Autodesk Inventor part; units mm, degrees
ref_plane "YZ Plane" through (0, 0, 0) normal (1, 0, 0) x (0, 1, 0)
ref_plane "XZ Plane" through (0, 0, 0) normal (0, 1, 0) x (-1, 0, 0)
ref_plane "XY Plane" through (0, 0, 0) normal (0, 0, 1) x (1, 0, 0)
sketch "Boceto1" plane through (0, 0, 0) normal (0, 1, 0) x (-1, 0, 0)
  circle A0 centre (22.76, 7.95) radius 1.5
  circle A1 centre (-26.24, 7.95) radius 1.5
  line L0 (29.635, -14.19) -> (29.635, 11.2)
  line L1 (29.635, 11.2) -> (-33.115, 11.2)
  line L2 (-33.115, 11.2) -> (-33.115, -14.19)
  line L3 (-33.115, -14.19) -> (29.635, -14.19)
  line L4 (-1.74, -3.0983) -> (-1.74, -1.495)
  line L5 (-1.74, -1.495) -> (-3.5727, -1.495)
  circle A2 centre (26.385, -10.94) radius 1.5
  circle A3 centre (-29.865, -10.94) radius 1.5
  circle A4 centre (26.385, 7.95) radius 1.5
  circle A5 centre (-29.865, 7.95) radius 1.5
  dimension "d5" = 25.39
  dimension "d6" = 62.75
  dimension "d7" = 3
  dimension "d8" = 3.25
  dimension "d9" = 3.25
  dimension "d10" = 49
  dimension "d11" = 0
  dimension "d24" = 3
extrude "Extrusión1" add sketch "Boceto1" along normal blind 3
sketch "Boceto2" plane through (0, 3, 0) normal (0, 1, 0) x (1, 0, 0)
  circle A0 centre (-26.385, -7.95) radius 1.5
  circle A1 centre (-26.385, -7.95) radius 2.5
  circle A2 centre (-26.385, 10.94) radius 1.5
  circle A3 centre (-26.385, 10.94) radius 2.5
  circle A4 centre (29.865, 10.94) radius 1.5
  circle A5 centre (29.865, 10.94) radius 2.5
  circle A6 centre (29.865, -7.95) radius 1.5
  circle A7 centre (29.865, -7.95) radius 2.5
  point P0 (0, 0)
  dimension "d14" = 5
  dimension "d15" = 5
  dimension "d16" = 5
  dimension "d17" = 5
extrude "Extrusión2" add sketch "Boceto2" along normal blind 3
sketch "Boceto3" plane through (0, 0, 0) normal (0, -1, 0) x (1, 0, 0)
  circle A0 centre (-22.76, 7.95) radius 1.5
  circle A1 centre (-22.76, 7.95) radius 3
  circle A2 centre (26.24, 7.95) radius 1.5
  circle A3 centre (26.24, 7.95) radius 3
  point P0 (0, 0)
  dimension "d20" = 6
  dimension "d21" = 6
extrude "Extrusión3" add sketch "Boceto3" along normal blind 15
properties part number "Soporte 16 pwm"
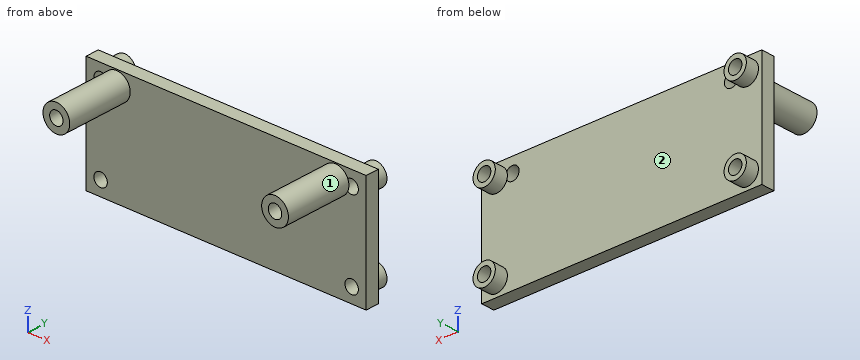
Could you check a few things on this model? Use its own coordinates, in mm. Face numbers are marked on the shaded views. A direction names the side the tool comes from. Round coordinates to 2 decimals unless told otherwise and drop trailing zeros. Write each loop counter-clockwise with the first axis right and the second up, starting at its lowest first coordinate (ties: lowest second). Pieces come first, ordered by that corner, then holes.
(1) Suppose I cut it at B-B on x = -22.76. Write out the boundary of the cut face in (y, z).
Findings below:
outline: (-15, 4.95) - (0, 4.95) - (0, -14.19) - (3, -14.19) - (3, 6.45) - (-15, 6.45) - close; (-15, 9.45) - (3, 9.45) - (3, 11.2) - (0, 11.2) - (0, 10.95) - (-15, 10.95) - close
(2) Suppose I cut it at C-C on y = -6.75. Write out the boundary of the cut face in (x, z).
Findings below:
outline: circle Ø6 at (-22.76, 7.95); circle Ø6 at (26.24, 7.95); hole circle Ø3 at (-22.76, 7.95); hole circle Ø3 at (26.24, 7.95)
(3) Suppose I cut it at A-A on y = 0.75. Write out the boundary of the cut face in (x, z) (3 decimals).
Findings below:
outline: (-29.635, -14.19) - (33.115, -14.19) - (33.115, 11.2) - (-29.635, 11.2) - close; hole circle Ø3 at (-26.385, -10.94); hole circle Ø3 at (-26.385, 7.95); hole circle Ø3 at (-22.76, 7.95); hole circle Ø3 at (26.24, 7.95); hole circle Ø3 at (29.865, -10.94); hole circle Ø3 at (29.865, 7.95)
(4) Suppose I cut it at D-D on z = -2.5. Write out the boundary of the cut face in (x, y) (3 decimals), and give its area (3 significant figures).
Findings below:
outline: (-29.635, 0) - (33.115, 0) - (33.115, 3) - (-29.635, 3) - close
area: 188 mm2
(5) Which directions (+Z, -Z, +X, -X, +Y, -Y) give clear straight access to the entire face, cutting with the end or side of a thin tool? Please do the marked faces 1 and 2.
Findings below:
face 1: -Y
face 2: +Y
(6) If I drill on probe 1 along X at (y, z) = (2.8, -10.94) (3 decimals); probe 2 along X at (y, z) = (2.45, 7.95) (3 decimals); probe 3 along Z at (x, y) = (26.24, 1.3), over which ranges is the centre line in solid material (lowest first)?
Findings below:
probe 1: x = -29.635 to -27.885, -24.885 to 28.365, 31.365 to 33.115
probe 2: x = -29.635 to -27.885, -24.885 to -24.26, -21.26 to 24.74, 27.74 to 28.365, 31.365 to 33.115
probe 3: z = -14.19 to 6.45, 9.45 to 11.2
(7) For pin 1 (4 mm diameter, centred on x = -22.76, z = 7.95, fed in from +Y); pin 2 (5 mm diameter, centred on x = 21, y = -7.5, fed in from +Z); pin 3 (1 mm diameter, centred on x = 29, z = 8, fed in from +Y); pin 4 (2 mm diameter, centred on x = 20, z = -10, fed in from -Y), each with a flat end and sliding along its axis, tell me the tip position at first contact or that it passes through.
Findings below:
pin 1: stops at y = 6
pin 2: stops at z = 9.17
pin 3: stops at y = 0
pin 4: stops at y = 0
